The model under review builds one solid part; all positions refer to its coordinate system, in mm. Face numbers are marked on the shaded views. A direction names the side the tool comes from. Give positions to 0.01 mm unless a question says otherwise; leave off trailing zeros. Order: outer loops, then holes, each group sorted by start corner. A loop starts at its lowest first (then second) coordinate and runs counter-clockwise, first axis right, second up. Notation, with made-up numbers: M 60.5,21 L 85.5,21 A28 ccw 85.5,58 Z; hole C 24,68 d8. An arc over 180 degrees is marked long. One line per question, with ' | ' between items. Start each with the question number.
1. The part is to be moulded in two halves that separate along Y. For the marked faces 5, 6 and 7, say which applies: +Y half, -Y half, draft (parallel to the pull), parting line (faces both ways), or undercut.
2. Insertion check: P1, Ø0.9, axis at x = 0.5, z = 3.5, coming from the +Y side; P2, Ø1.5, axis at y = 0, z = 4.5, coming from the -X side; P3, Ø1, axis at x = -2.5, z = 1, coming from the -Y side. Each pin has a flat end and moves straight along its axis. Give the tip position at first contact, or say it passes through.
3. For the marked faces 1, 2, 3 and 4, list the 3-axis set-ups (+Z, -Z, +X, -X, +Y, -Y) from which the entire face can be reached by the end or side of a thin tool; tool diameter is ignored.
4. We need section D-D on y = -2.25. Write out the cut boundary in (x, z).
5. Wall thickness on L1, parallel to Y at x = 0, z = 1.75; L2, parallel to Y at x = 0, z = 2.75: over which ranges is each line inside the solid? List them lowest first.
6. We need section B-B on y = 0. Write out the cut boundary in (x, z), then the cut area to 3 significant figures.
7. We need section A-A on z = 5. Write out the cut boundary in (x, y).
```python
from build123d import *

# Parameters (mm, degrees)
SKETCH1_R           = 4.1
BOSS_EXTRUDE1_DEPTH = 2.5
SKETCH2_W           = 5.2
SKETCH2_H           = 5.2
BOSS_EXTRUDE2_DEPTH = 4
SKETCH3_R           = 2.1
CUT_EXTRUDE1_DEPTH  = 9.710338685
FILLET1_R           = 1


with BuildPart() as part:
    # Sketch1 → Boss-Extrude1 (new body)
    with BuildSketch(Plane(origin=(0, 0, 0), x_dir=(0, 1, 0), z_dir=(0, 0, 1))):
        with Locations(Location((0, 0, 0), (0, 0, 270))):
            Circle(SKETCH1_R)
    extrude(amount=BOSS_EXTRUDE1_DEPTH)

    # Sketch2 → Boss-Extrude2 (add)
    with BuildSketch(Plane.XY.offset(2.5)):
        Rectangle(SKETCH2_W, SKETCH2_H)
    extrude(amount=BOSS_EXTRUDE2_DEPTH)

    # Sketch3 → Cut-Extrude1 (cut, through all)
    with BuildSketch(Plane.XY.offset(6.5)):
        Circle(SKETCH3_R)
    extrude(amount=-CUT_EXTRUDE1_DEPTH, mode=Mode.SUBTRACT)

    # Fillet1
    # the kernel refuses this fillet: 1 mm, written as the material it takes off along each edge
    with BuildSketch(Plane(origin=(-1.6, -1.6, 5.5), x_dir=(0, -1, 0), z_dir=(0, 0, 1))) as fillet1_piece_1_section:
        Polygon((0, 0), (FILLET1_R, 0), (FILLET1_R, -FILLET1_R), (0, -FILLET1_R), align=None)
    fillet1_piece_1 = extrude(amount=FILLET1_R, mode=Mode.PRIVATE)
    fillet1_piece_1 = fillet1_piece_1 - Plane(origin=(-1.6, -1.6, 5.5), x_dir=(0.7071067811865475, 0.7071067811865475, 0), z_dir=(0, 0, 1)) * Sphere(FILLET1_R, mode=Mode.PRIVATE)
    add(fillet1_piece_1, mode=Mode.SUBTRACT)
    with BuildSketch(Plane(origin=(1.6, -1.6, 5.5), x_dir=(0, -1, 0), z_dir=(0, 0, 1))) as fillet1_piece_2_section:
        Polygon((0, 0), (FILLET1_R, 0), (FILLET1_R, FILLET1_R), (0, FILLET1_R), align=None)
    fillet1_piece_2 = extrude(amount=FILLET1_R, mode=Mode.PRIVATE)
    fillet1_piece_2 = fillet1_piece_2 - Plane(origin=(1.6, -1.6, 5.5), x_dir=(-0.7071067811865475, 0.7071067811865475, 0), z_dir=(0, 0, 1)) * Sphere(FILLET1_R, mode=Mode.PRIVATE)
    add(fillet1_piece_2, mode=Mode.SUBTRACT)
    with BuildSketch(Plane(origin=(1.6, 1.6, 5.5), x_dir=(1, 0, 0), z_dir=(0, 0, 1))) as fillet1_piece_3_section:
        Polygon((0, 0), (FILLET1_R, 0), (FILLET1_R, FILLET1_R), (0, FILLET1_R), align=None)
    fillet1_piece_3 = extrude(amount=FILLET1_R, mode=Mode.PRIVATE)
    fillet1_piece_3 = fillet1_piece_3 - Plane(origin=(1.6, 1.6, 5.5), x_dir=(-0.7071067811865475, -0.7071067811865475, 0), z_dir=(0, 0, 1)) * Sphere(FILLET1_R, mode=Mode.PRIVATE)
    add(fillet1_piece_3, mode=Mode.SUBTRACT)
    with BuildSketch(Plane(origin=(-1.6, 1.6, 5.5), x_dir=(0, 1, 0), z_dir=(0, 0, 1))) as fillet1_piece_4_section:
        Polygon((0, 0), (FILLET1_R, 0), (FILLET1_R, FILLET1_R), (0, FILLET1_R), align=None)
    fillet1_piece_4 = extrude(amount=FILLET1_R, mode=Mode.PRIVATE)
    fillet1_piece_4 = fillet1_piece_4 - Plane(origin=(-1.6, 1.6, 5.5), x_dir=(0.7071067811865475, -0.7071067811865475, 0), z_dir=(0, 0, 1)) * Sphere(FILLET1_R, mode=Mode.PRIVATE)
    add(fillet1_piece_4, mode=Mode.SUBTRACT)
    with BuildSketch(Plane(origin=(-1.6, -2.6, 6.5), x_dir=(0, 0, -1), z_dir=(1, 0, 0)), Plane(origin=(2.6, -1.6, 6.5), x_dir=(0, 0, -1), z_dir=(0, 1, 0)), Plane(origin=(1.6, 2.6, 6.5), x_dir=(0, 0, -1), z_dir=(-1, 0, 0)), Plane(origin=(-2.6, 1.6, 6.5), x_dir=(0, 0, -1), z_dir=(0, -1, 0))) as fillet1_piece_5:
        with BuildLine():
            CenterArc((FILLET1_R, FILLET1_R), FILLET1_R, 180, 90)
            Line((0, FILLET1_R), (0, 0))
            Line((0, 0), (FILLET1_R, 0))
        make_face()
    extrude(amount=3.2, mode=Mode.SUBTRACT)
    with BuildSketch(Plane(origin=(2.6, -2.6, 2.5), x_dir=(-1, 0, 0), z_dir=(0, 0, 1)), Plane(origin=(2.6, 2.6, 2.5), x_dir=(0, -1, 0), z_dir=(0, 0, 1)), Plane(origin=(-2.6, 2.6, 2.5), x_dir=(1, 0, 0), z_dir=(0, 0, 1))) as fillet1_piece_6:
        with BuildLine():
            CenterArc((FILLET1_R, -FILLET1_R), FILLET1_R, 90, 90)
            Line((0, -FILLET1_R), (0, 0))
            Line((0, 0), (FILLET1_R, 0))
        make_face()
    extrude(amount=3, mode=Mode.SUBTRACT)
    with BuildSketch(Plane(origin=(-2.6, -2.6, 2.5), x_dir=(1, 0, 0), z_dir=(0, 0, 1))) as fillet1_piece_7:
        with BuildLine():
            CenterArc((FILLET1_R, FILLET1_R), FILLET1_R, 180, 90)
            Line((0, FILLET1_R), (0, 0))
            Line((0, 0), (FILLET1_R, 0))
        make_face()
    extrude(amount=3, mode=Mode.SUBTRACT)


solid = part.part
```
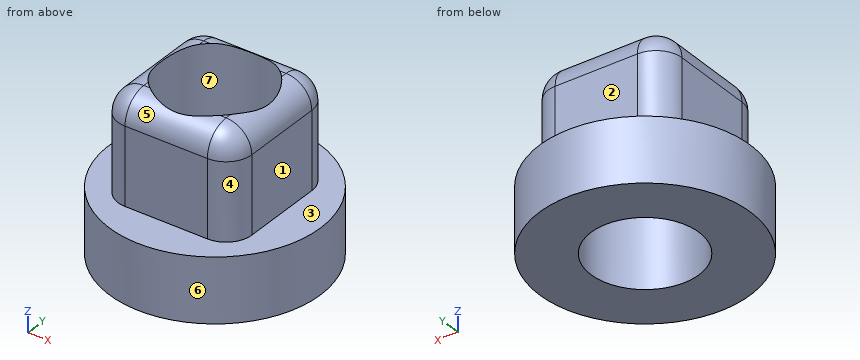
Entries:
1) face 5: -Y half | face 6: parting line | face 7: undercut
2) P1: stops at y = 2.6 | P2: stops at x = -2.6 | P3: stops at y = -3.58
3) face 1: +Z, +X, +Y, -Y | face 2: +Z, +X, -X, +Y | face 3: +Z | face 4: +Z, +X, -Y
4) outline: M -3.43,0 L 3.43,0 L 3.43,2.5 L 2.36,2.5 L 2.36,5.5 A0.76 ccw 1.6,6.26 L -1.6,6.26 A0.76 ccw -2.36,5.5 L -2.36,2.5 L -3.43,2.5 Z
5) L1: y = -4.1 to -2.1, 2.1 to 4.1 | L2: y = -2.6 to -2.1, 2.1 to 2.6
6) outline: M -4.1,0 L -2.1,0 L -2.1,6.37 A1 ccw -2.6,5.5 L -2.6,2.5 L -4.1,2.5 Z; M 2.1,0 L 4.1,0 L 4.1,2.5 L 2.6,2.5 L 2.6,5.5 A1 ccw 2.1,6.37 Z | area: 13.6 mm^2
7) outline: M -2.6,-1.6 A1 ccw -1.6,-2.6 L 1.6,-2.6 A1 ccw 2.6,-1.6 L 2.6,1.6 A1 ccw 1.6,2.6 L -1.6,2.6 A1 ccw -2.6,1.6 Z; hole C 0,0 d4.2
